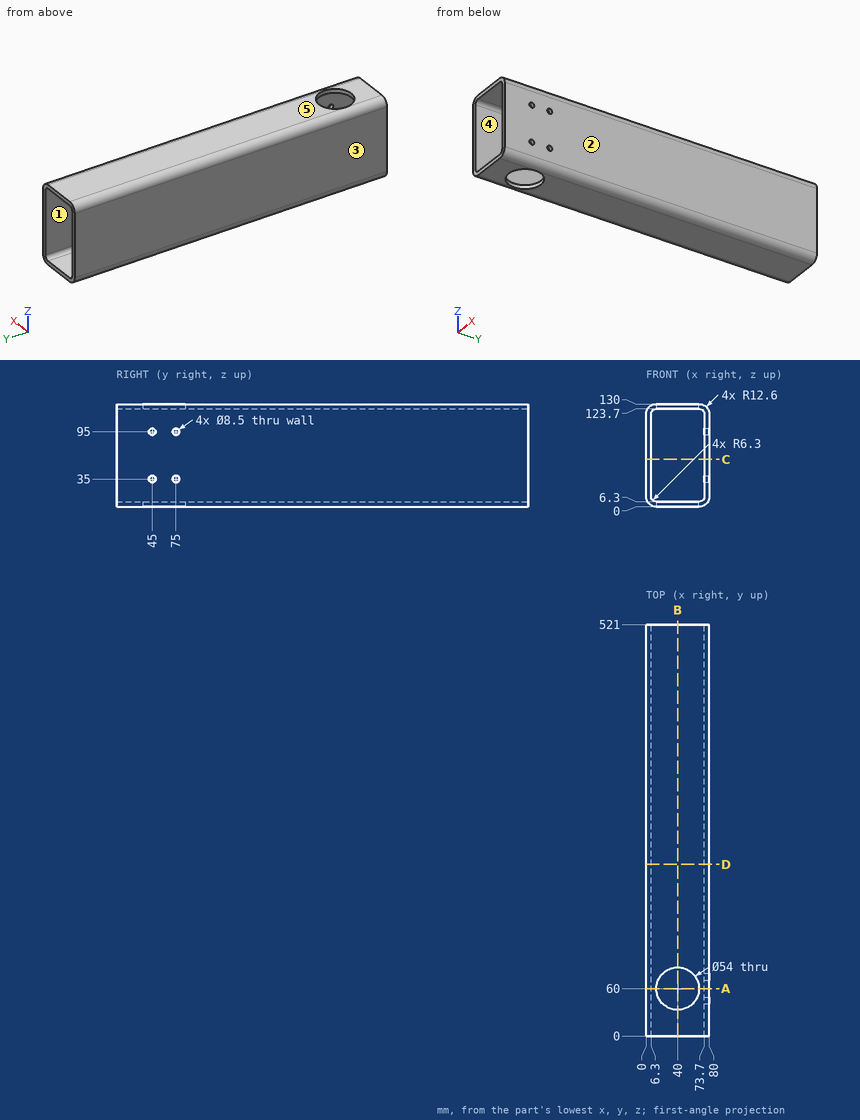
Check sheet for the drawn part. Datum: minimum x, y, z corner. Units: mm. A direction names the side the tool comes from. Coordinates: 2 decimals unless noted, no trailing zeros. Write each loop counter-clockwise with the first axis right and the second up, starting at its lowest first coordinate (ties: lowest second). Pieces come first, ordered by that corner, then holes. Notation, with made-up numbers: M 9,50.5 L 65,50.5 A19 cw 65,65.5 Z; hole C -6,47.5 d1. An arc over 180 degrees is marked long. One line per item, written item: value.
Item 1: Scan lines: line 1 along Y through (x, z) = (77.25, 95); line 2 along Z through (x, y) = (58.5, 327); line 3 along Z through (x, y) = (76, 45). Record each from-to range of solid material in increasing order.
Check sheet entries:
line 1: y = 0 to 40.75, 49.25 to 70.75, 79.25 to 521
line 2: z = 0 to 6.3, 123.7 to 130
line 3: z = 3.39 to 30.75, 39.25 to 90.75, 99.25 to 126.61
Item 2: Gauge pin test, flat ends, axial feed: pin 1 Ø7 at (y, z) = (75, 35) entering from +X; pin 2 Ø5 at (x, y) = (70.5, 431.5) entering from +Z. Record the tip position at first contact, or that the pin passes through.
Check sheet entries:
pin 1: stops at x = 6.3
pin 2: stops at z = 129.99
Item 3: Mould release check, pull along X, two halves, no side actions. Record for the marked faces 3, 4 and 5: pulls with the +X half, pulls with the -X half, needs draft (parallel to the pull), parting line crosses it, or undercut.
Check sheet entries:
face 3: pulls with the -X half
face 4: undercut
face 5: needs draft
Item 4: Section check A-A, the plane y = 60. Record the boundary of the cut face in (x, z), plus the area to 3 significant figures.
Check sheet entries:
outline: M 0,12.6 A12.6 ccw 12.6,0 L 13,0 L 13,6.3 L 12.6,6.3 A6.3 cw 6.3,12.6 L 6.3,117.4 A6.3 cw 12.6,123.7 L 13,123.7 L 13,130 L 12.6,130 A12.6 ccw 0,117.4 Z; M 67,0 L 67.4,0 A12.6 ccw 80,12.6 L 80,117.4 A12.6 ccw 67.4,130 L 67,130 L 67,123.7 L 67.4,123.7 A6.3 cw 73.7,117.4 L 73.7,12.6 A6.3 cw 67.4,6.3 L 67,6.3 Z
area: 1,700 mm^2
Item 5: Access from +Z, -Z, +X, -X, +Y, -Y to the whole of each face (thin tool, end or side, straight path). Record for the marked faces 1 and 2.
Check sheet entries:
face 1: +Y, -Y
face 2: +Z, -Z, +X, +Y, -Y
Item 6: Section check B-B, the plane x = 40. Record the boundary of the cut face in (y, z), plus the area to 3 significant figures.
Check sheet entries:
outline: M 0,0 L 33,0 L 33,6.3 L 0,6.3 Z; M 0,123.7 L 33,123.7 L 33,130 L 0,130 Z; M 87,0 L 521,0 L 521,6.3 L 87,6.3 Z; M 87,123.7 L 521,123.7 L 521,130 L 87,130 Z
area: 5,880 mm^2
Item 7: Section check D-D, the plane y = 217.5. Record the boundary of the cut face in (x, z), plus the area to 3 significant figures.
Check sheet entries:
outline: M 0,12.6 A12.6 ccw 12.6,0 L 67.4,0 A12.6 ccw 80,12.6 L 80,117.4 A12.6 ccw 67.4,130 L 12.6,130 A12.6 ccw 0,117.4 Z; hole M 6.3,12.6 A6.3 ccw 12.6,6.3 L 67.4,6.3 A6.3 ccw 73.7,12.6 L 73.7,117.4 A6.3 ccw 67.4,123.7 L 12.6,123.7 A6.3 ccw 6.3,117.4 Z
area: 2,390 mm^2
Item 8: Section check C-C, the plane z = 60. Record the boundary of the cut face in (x, y), plus the area to 3 significant figures.
Check sheet entries:
outline: M 0,0 L 6.3,0 L 6.3,521 L 0,521 Z; M 73.7,0 L 80,0 L 80,521 L 73.7,521 Z
area: 6,560 mm^2
